Check sheet for the modelled part. Datum: model origin and axes. Units: mm. Face numbers are marked on the shaded views. Coordinates: 2 decimals unless noted, no trailing zeros. Order: outer loops, then holes, each group sorted by start corner. A loop starts at its lowest first (then second) coordinate and runs counter-clockwise, first axis right, second up.
1. Cross-section at D-D (z = -2.8). Enter the section's corners in (x, y), then the cut area to 3 significant figures.
2. Gauge pin test, flat ends, axial feed: pin 1 Ø1.5 at (y, z) = (2, -20) entering from +X; pin 2 Ø1.5 at (x, y) = (18.5, 1.5) entering from +Z; pin 3 Ø0.9 at (x, y) = (16.5, 1.5) entering from -Z. Record the tip position at first contact, or that the pin passes through.
3. Cross-section at B-B (z = 3.7). Enter the section's corners in (x, y).
4. Draft check along X on the marked faces 1 and 2. Enter one of: released by +X, released by -X, zero draft, split by the parting line, or undercut.
5. Cross-section at C-C (y = 2.1). Enter the section's corners in (x, z).
6. Thickness scan on line 1 (Z direction, x = 5, y = 1.25); line 2 (Z direction, x = 11.5, y = 1.9); line 3 (Z direction, x = 1, y = 0.9). Record the ranges inside material, lowest first.
7. Cross-section at A-A (x = 5). Enter the section's corners in (y, z).
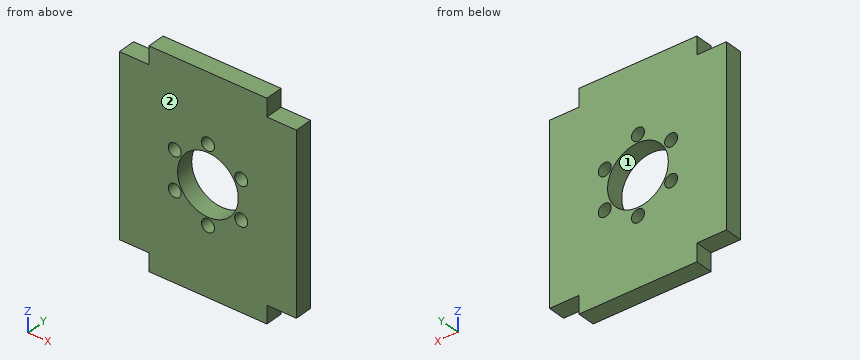
Autodesk Inventor part; units mm, degrees
ref_plane "YZ Plane" through (0, 0, 0) normal (1, 0, 0) x (0, 1, 0)
ref_plane "XZ Plane" through (0, 0, 0) normal (0, 1, 0) x (-1, 0, 0)
ref_plane "XY Plane" through (0, 0, 0) normal (0, 0, 1) x (1, 0, 0)
sketch "Sketch1" plane through (0, 0, 0) normal (0, 1, 0) x (-1, 0, 0)
  circle A0 centre (-5, -2.8) radius 5.15
  line L0 (10, -17.8) -> (10, 12.2)
  line L1 (-20, -17.8) -> (-20, 12.2)
  line L2 (10, 12.2) -> (5, 12.2)
  line L3 (5, 12.2) -> (5, 15.2)
  line L4 (-15, 15.2) -> (-15, 12.2)
  circle A1 centre (-5, 3.7) radius 1.1
  circle A2 centre (-10.6292, 0.45) radius 1.1
  circle A3 centre (-10.6292, -6.05) radius 1.1
  circle A4 centre (-5, -9.3) radius 1.1
  circle A5 centre (0.6292, -6.05) radius 1.1
  circle A6 centre (0.6292, 0.45) radius 1.1
  line L5 (-15, 12.2) -> (-20, 12.2)
  line L6 (5, 15.2) -> (-15, 15.2)
  line L7 (10, -17.8) -> (5, -17.8)
  line L8 (5, -17.8) -> (5, -20.8)
  line L9 (5, -20.8) -> (-15, -20.8)
  line L10 (-15, -20.8) -> (-15, -17.8)
  line L11 (-15, -17.8) -> (-20, -17.8)
  line L12 (-20, -17.8) -> (-20, -2.8)
  line L13 (-20, -2.8) -> (-5, -2.8)
  dimension "d7" = 360
  dimension "d42" = 30
  dimension "d43" = 5
  dimension "d44" = 3
  dimension "d49" = 2.2
  dimension "d52" = 360
  dimension "d57" = 30
  dimension "d59" = 5
  dimension "d60" = 3
  dimension "d61" = 20
  dimension "d62" = 15
extrude "Extrusion1" add sketch "Sketch1" along normal blind 3
properties part number "Motor Mount" material "PVC, Unplasticized"
Data:
1. outline: (-10, 0) - (-0.15, 0) - (-0.15, 3) - (-10, 3) - close; (10.15, 0) - (20, 0) - (20, 3) - (10.15, 3) - close
1. area: 59.1 mm2
2. pin 1: stops at x = 15
2. pin 2: stops at z = 12.2
2. pin 3: stops at z = -17.8
3. outline: (-10, 0) - (3.9, 0) - (3.9, 3) - (-10, 3) - close; (6.1, 0) - (20, 0) - (20, 3) - (6.1, 3) - close
4. face 1: undercut
4. face 2: zero draft
5. outline: (-10, -17.8) - (-5, -17.8) - (-5, -20.8) - (15, -20.8) - (15, -17.8) - (20, -17.8) - (20, 12.2) - (15, 12.2) - (15, 15.2) - (-5, 15.2) - (-5, 12.2) - (-10, 12.2) - close; hole circle Ø2.2 at (-0.63, -6.05); hole circle Ø2.2 at (-0.63, 0.45); hole circle Ø10.3 at (5, -2.8); hole circle Ø2.2 at (5, -9.3); hole circle Ø2.2 at (5, 3.7); hole circle Ø2.2 at (10.63, -6.05); hole circle Ø2.2 at (10.63, 0.45)
6. line 1: z = -20.8 to -10.4, -8.2 to -7.95, 2.35 to 2.6, 4.8 to 15.2
6. line 2: z = -20.8 to -6.72, -5.38 to -0.22, 1.12 to 15.2
6. line 3: z = -20.8 to -6.04, 0.44 to 15.2
7. outline: (0, -20.8) - (3, -20.8) - (3, -10.4) - (0, -10.4) - close; (0, -8.2) - (3, -8.2) - (3, -7.95) - (0, -7.95) - close; (0, 2.35) - (3, 2.35) - (3, 2.6) - (0, 2.6) - close; (0, 4.8) - (3, 4.8) - (3, 15.2) - (0, 15.2) - close
